Verification items for the finished model (mm, model axes). A direction names the side the tool comes from. Round coordinates to 2 decimals unless told otherwise and drop trailing zeros. Loops run counter-clockwise (first coordinate to the right, second up) from the corner with the lowest first, then second, coordinate; pieces in that order, holes last. Notation, with made-up numbers: (-23, 67) - (-19, 67) arc R25 cw to (-19, 86) - close; hole circle Ø5 at (58, 26.5). An arc over 180 degrees is marked (long way). Use CSV: the item, a comma, the result in double quotes.
```python
from build123d import *

# Parameters (mm, degrees)
SKETCH_1_R      = 30
EXTRUDE_1_DEPTH = 6
EXTRUDE_2_DEPTH = 50


with BuildPart() as part:
    # 草图1 → 凸台-拉伸1 (new body)
    with BuildSketch(Plane.XY):
        with BuildLine():
            Line((60, 50), (0, 50))
            Line((0, 50), (0, -50))
            Line((0, -50), (60, -50))
            ThreePointArc((60, -50), (110, 0), (60, 50))
        make_face()
        with Locations((60, 0)):
            Circle(SKETCH_1_R, mode=Mode.SUBTRACT)
    extrude(amount=EXTRUDE_1_DEPTH)

    # 草图2 → 凸台-拉伸2 (add, symmetric)
    with BuildSketch(Plane(origin=(0, 0, 0), x_dir=(1, 0, 0), z_dir=(0, 1, 0))):
        Polygon((0, 0), (0, 30), (-40, 30), (-40, 36), (6, 36), (6, 0), align=None)
    extrude(amount=EXTRUDE_2_DEPTH, both=True)


solid = part.part
```
1) Access from +Z, -Z, +X, -X, +Y, -Y to the whole of each face (thin tool, end or side, straight path). Record for faces 5 (the face through (109.988, -1.099, 2.958)), 6 (the face through (34, 23, 0)), 7 (the face through (-20, 1, -30)).
Returned:
face 5,"+Z, -Z, +X"
face 6,"-Z, +X, +Y, -Y"
face 7,"+Z, -X, +Y, -Y"
2) Cross-section at D-D, the plane y = 41. Record the cut outline in (x, z), then the cut area to 3 significant figures.
Returned:
outline,"(-40, -36) - (6, -36) - (6, 0) - (88.62, 0) - (88.62, 6) - (0, 6) - (0, -30) - (-40, -30) - close"
area,"988 mm²"
3) Mould release check, pull along X, two halves, no side actions. Record for faces 1 (the face through (30.03, 1.32, 2.96)), 2 (the face through (6, 1, -18)), 3 (the face through (3, -50, -12)), 4 (the face through (-40, 1, -33)): +X half, -X half, draft (parallel to the pull), parting line (faces both ways), or undercut.
Returned:
face 1,"undercut"
face 2,"+X half"
face 3,"draft"
face 4,"-X half"
4) Cross-section at A-A, the plane z = 3. Record the cut outline in (x, y).
Returned:
outline,"(0, -50) - (60, -50) arc R50 ccw to (60, 50) - (0, 50) - close; hole circle Ø60 at (60, 0)"
5) Cross-section at B-B, the plane x = 47. Record the cut outline in (y, z).
Returned:
outline,"(-50, 0) - (-27.04, 0) - (-27.04, 6) - (-50, 6) - close; (27.04, 0) - (50, 0) - (50, 6) - (27.04, 6) - close"
6) Gauge pin test, flat ends, axial feed: pin 1 Ø11 at (y, z) = (17.5, -20) entering from +X; pin 2 Ø6 at (x, y) = (93, 37) entering from -Z; pin 3 Ø5 at (y, z) = (-17, -6.5) entering from -X. Record the tip position at first contact, or that the pin passes through.
Returned:
pin 1,"stops at x = 6"
pin 2,"stops at z = 0"
pin 3,"stops at x = 0"
7) Cross-section at C-C, the plane y = -7.5. Record the cut outline in (x, z).
Returned:
outline,"(-40, -36) - (6, -36) - (6, 0) - (30.95, 0) - (30.95, 6) - (0, 6) - (0, -30) - (-40, -30) - close; (89.05, 0) - (109.43, 0) - (109.43, 6) - (89.05, 6) - close"
8) Thickness scan on probe 1 along Y at (x, z) = (60, 1.65); probe 2 along Z at (x, y) = (-1, 6); probe 3 along X at (y, z) = (-38.5, -16.5). Record the ranges inside material, lowest first. Write a range as [from, to].
Returned:
probe 1,"y = [-50, -30], [30, 50]"
probe 2,"z = [-36, -30]"
probe 3,"x = [0, 6]"
